Design review of the part built by this model. Coordinates are the model's own, in mm. Face numbers are marked on the shaded views. A direction names the side the tool comes from. Give positions to 0.01 mm unless a question says otherwise; leave off trailing zeros. Order: outer loops, then holes, each group sorted by start corner. A loop starts at its lowest first (then second) coordinate and runs counter-clockwise, first axis right, second up.
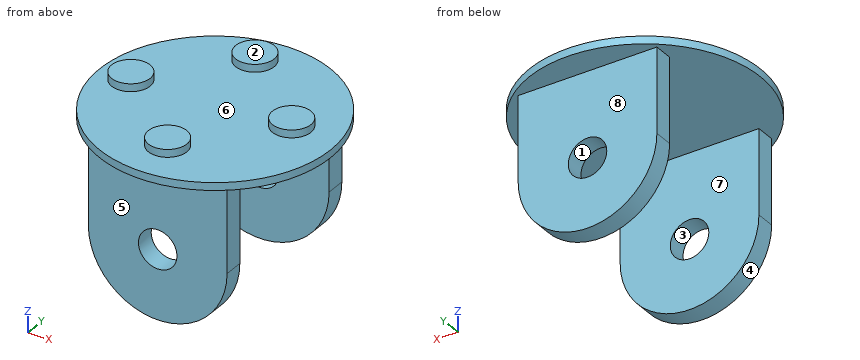
```python
from build123d import *

# Parameters (mm, degrees)
SKETCH1_R           = 30
BOSS_EXTRUDE1_DEPTH = 2
SKETCH3_W           = 36
SKETCH3_H           = 5
BOSS_EXTRUDE3_DEPTH = 22
BOSS_EXTRUDE4_DEPTH = 5
SKETCH6_R           = 5
CUT_EXTRUDE1_DEPTH  = 22
SKETCH7_R           = 5
BOSS_EXTRUDE5_DEPTH = 2


with BuildPart() as part:
    # Sketch1 → Boss-Extrude1 (new body)
    with BuildSketch(Plane.XY):
        Circle(SKETCH1_R)
    extrude(amount=-BOSS_EXTRUDE1_DEPTH)

    # Sketch3 → Boss-Extrude3 (add)
    with BuildSketch(Plane(origin=(0, 0, -2), x_dir=(-1, 0, 0), z_dir=(0, 0, -1))):
        with Locations((0, -20)):
            Rectangle(SKETCH3_W, SKETCH3_H)
    boss_extrude3 = extrude(amount=BOSS_EXTRUDE3_DEPTH)

    # Sketch5 → Boss-Extrude4 (add)
    with BuildSketch(Plane.XZ.offset(22.5)):
        with BuildLine():
            Line((-18, -24), (18, -24))
            ThreePointArc((18, -24), (0, -42), (-18, -24))
        make_face()
    boss_extrude4 = extrude(amount=-BOSS_EXTRUDE4_DEPTH)

    # Sketch6 → Cut-Extrude1 (cut)
    with BuildSketch(Plane(origin=(0, -17.5, 0), x_dir=(1, 0, 0), z_dir=(0, 1, 0))):
        with Locations(Location((0, 24, 0), (0, 0, 180))):
            Circle(SKETCH6_R)
    cut_extrude1 = extrude(amount=-CUT_EXTRUDE1_DEPTH, mode=Mode.SUBTRACT)

    # Mirror2: Boss-Extrude3, Boss-Extrude4, Cut-Extrude1 across plane
    add(boss_extrude3.mirror(Plane.ZX))
    add(boss_extrude4.mirror(Plane.ZX))
    add(cut_extrude1.mirror(Plane.ZX), mode=Mode.SUBTRACT)

    # Sketch7 → Boss-Extrude5 (add)
    with BuildSketch(Plane.XY):
        with Locations((-3.94, 21.58)):
            Circle(SKETCH7_R)
        with Locations((-21.94, 0.13)):
            Circle(SKETCH7_R)
        with Locations((-0.49, -17.87)):
            Circle(SKETCH7_R)
        with Locations((17.51, 3.58)):
            Circle(SKETCH7_R)
    extrude(amount=BOSS_EXTRUDE5_DEPTH)


solid = part.part
```
1. Draft analysis for pull direction Z (two halves, no side actions). For the marked faces 1, 2, 3 and 4, state which applies: pulls with the +Z half, pulls with the -Z half, needs draft (parallel to the pull), parting line crosses it, or undercut.
Recorded:
face 1: undercut
face 2: pulls with the +Z half
face 3: undercut
face 4: pulls with the -Z half
2. Take a section at A-A (z = -8). State the section outline as (x, y) points.
Recorded:
outline: (-18, -22.5) - (18, -22.5) - (18, -17.5) - (-18, -17.5) - close; (-18, 17.5) - (18, 17.5) - (18, 22.5) - (-18, 22.5) - close
3. Machinability: for the marked faces 5, 6, 7 and 8, which of the approach directions +Z, -Z, +X, -X, +Y, -Y give a long, thin tool a straight path to every point of the face, cutting with its end or side? Answer none if there is none.
Recorded:
face 5: -Z, +X, -X, -Y
face 6: +Z
face 7: -Z, +X, -X
face 8: -Z, +X, -X, +Y
4. Take a section at B-B (x = -0.49). State the section outline as (y, z) points, then the cut area to 3 significant figures.
Recorded:
outline: (-30, -2) - (-22.5, -2) - (-22.5, -19.02) - (-17.5, -19.02) - (-17.5, -2) - (17.5, -2) - (17.5, -19.02) - (22.5, -19.02) - (22.5, -2) - (30, -2) - (30, 0) - (25.2, 0) - (25.2, 2) - (17.96, 2) - (17.96, 0) - (-12.87, 0) - (-12.87, 2) - (-22.87, 2) - (-22.87, 0) - (-30, 0) - close; (-22.5, -41.99) - (-17.5, -41.99) - (-17.5, -28.98) - (-22.5, -28.98) - close; (17.5, -41.99) - (22.5, -41.99) - (22.5, -28.98) - (17.5, -28.98) - close
area: 455 mm2
5. For pin 1 (11 mm diameter, centred on x = -7, z = -29.5, fed in from -Y); pin 2 (16 mm diameter, centred on x = 0, z = -24, fed in from +Y); pin 3 (4 mm diameter, centred on y = -19.5, z = -16.5, fed in from -X), all flat-tipped, find the tip position at first contact; note any pin that passes through.
Recorded:
pin 1: stops at y = -22.5
pin 2: stops at y = 22.5
pin 3: stops at x = -18
6. Take a section at C-C (z = -28). State the section outline as (x, y) points, then the cut area to 3 significant figures.
Recorded:
outline: (-17.55, -22.5) - (-3, -22.5) - (-3, -17.5) - (-17.55, -17.5) - close; (-17.55, 17.5) - (-3, 17.5) - (-3, 22.5) - (-17.55, 22.5) - close; (3, -22.5) - (17.55, -22.5) - (17.55, -17.5) - (3, -17.5) - close; (3, 17.5) - (17.55, 17.5) - (17.55, 22.5) - (3, 22.5) - close
area: 291 mm2
7. Take a section at D-D (y = 3.58). State the section outline as (x, z) points.
Recorded:
outline: (-29.79, -2) - (29.79, -2) - (29.79, 0) - (22.51, 0) - (22.51, 2) - (12.51, 2) - (12.51, 0) - (-18.32, 0) - (-18.32, 2) - (-25.56, 2) - (-25.56, 0) - (-29.79, 0) - close
8. For line 1 along Y through (x, z) = (14.5, -34); line 2 along X through (y, z) = (20.5, -24); line 3 along Z through (x, y) = (0, -20), list the stretches that pass through material, from the lowest coordinate up.
Recorded:
line 1: y = -22.5 to -17.5, 17.5 to 22.5
line 2: x = -18 to -5, 5 to 18
line 3: z = -42 to -29, -19 to 2
